Autodesk Inventor part; units mm, degrees
ref_plane "YZ Plane" through (0, 0, 0) normal (1, 0, 0) x (0, 1, 0)
ref_plane "XZ Plane" through (0, 0, 0) normal (0, 1, 0) x (-1, 0, 0)
ref_plane "XY Plane" through (0, 0, 0) normal (0, 0, 1) x (1, 0, 0)
sketch "Sketch1" plane through (0, 0, 0) normal (1, 0, 0) x (0, 1, 0)
  line L0 (0, 0) -> (17.9, 0)
  line L1 (17.9, 0) -> (17.9, 85)
  line L2 (17.9, 85) -> (0, 85)
  line L3 (0, 85) -> (0, 0)
  dimension "d0" = 17.9
  dimension "d1" = 85
extrude "Extrusion1" add sketch "Sketch1" along normal blind 10
fillet "Fillet1" radius 8.95 2 edges at (5, 17.9, 85) (5, 0, 85)
sketch "Sketch2" plane through (10, 0, 0) normal (1, 0, 0) x (0, 0, -1)
  arc A0 (-76.05, 17.9) -> (-76.05, 0) centre (-76.05, 8.95) ccw
  circle A1 centre (-76.05, 8.95) radius 4.75
  point P0 (0, 0)
  dimension "d5" = 9.5
extrude "Extrusion2" cut sketch "Sketch2" against normal blind 10
sketch "Sketch3" plane through (0, 0, 0) normal (0, 0, -1) x (-1, 0, 0)
  line L0 (14.8, 0) -> (-24.8, 0)
  line L1 (-31.8, 7) -> (-31.8, 7)
  line L2 (-24.8, 14) -> (14.8, 14)
  line L3 (21.8, 7) -> (21.8, 7)
  line L4 (0, 0) -> (0, 17.9)
  line L5 (-10, 0) -> (-10, 17.9)
  line L6 (0, 17.9) -> (-10, 17.9)
  circle A0 centre (-25.7, 7) radius 1.6
  circle A1 centre (15.7, 7) radius 1.6
  arc A2 (-24.8, 14) -> (-31.8, 7) centre (-24.8, 7) ccw
  arc A3 (-31.8, 7) -> (-24.8, 0) centre (-24.8, 7) ccw
  arc A4 (21.8, 7) -> (14.8, 14) centre (14.8, 7) ccw
  arc A5 (14.8, 0) -> (21.8, 7) centre (14.8, 7) ccw
  point P0 (21.8, 0)
  point P1 (-31.8, 14)
  point P2 (-31.8, 0)
  point P3 (21.8, 14)
  point P4 (-10, 14)
  point P5 (0, 14)
  point P6 (21.8, 7)
  point P7 (-31.8, 7)
  dimension "d8" = 14
  dimension "d9" = 21.8
  dimension "d10" = 21.8
  dimension "d11" = 17.9
  dimension "d12" = 3.2
  dimension "d13" = 3.2
  dimension "d14" = 6.1
  dimension "d15" = 6.1
  dimension "d16" = 7
  dimension "d17" = 7
  dimension "d23" = 7
extrude "Extrusion3" add sketch "Sketch3" against normal blind 10 contours L0 L4 L2 A4 A5 | L0 L5 L2 L4 | L0 A3 A2 L2 L5
fillet "Fillet3" radius 5.5 2 edges at (10, 7, 10) (0, 7, 10)
fillet "Fillet4" radius 3.9 4 edges at (0, 14, 12.75) (0, 14, 5) (10, 14, 12.75) (10, 14, 5)
sketch "Sketch4" plane through (24.8, 7, 0) normal (0, 0, -1) x (-1, 0, 0)
  line L0 (14.8, 10.9) -> (14.8, -7)
  line L1 (14.8, 10.9) -> (24.8, 10.9)
  line L2 (24.8, 10.9) -> (24.8, 14.4)
  line L3 (19.8, 19.4) -> (19.8, 19.4)
  line L4 (14.8, 14.4) -> (14.8, 10.9)
  circle A0 centre (19.8, 15.7) radius 1.6
  arc A1 (19.8, 19.4) -> (14.8, 14.4) centre (19.8, 14.4) ccw
  arc A2 (24.8, 14.4) -> (19.8, 19.4) centre (19.8, 14.4) ccw
  point P0 (24.8, -7)
  point P1 (24.8, 19.4)
  point P2 (19.8, 19.4)
  dimension "d24" = 8.5
  dimension "d25" = 3.2
  dimension "d26" = 4.8
  dimension "d27" = 5
extrude "Extrusion4" add sketch "Sketch4" against normal blind 10
fillet "Fillet5" radius 3 1 edges at (5, 17.9, 10)
properties part number "Motor Mount V2"
Verification items for the finished model (mm, model axes). A direction names the side the tool comes from. Round coordinates to 2 decimals unless told otherwise and drop trailing zeros. Loops run counter-clockwise (first coordinate to the right, second up) from the corner with the lowest first, then second, coordinate; pieces in that order, holes last. Notation, with made-up numbers: (63.5, 81.25) - (84.5, 81.25) arc R22 ccw to (84.5, 91.25) - close; hole circle Ø5 at (75, 4). An arc over 180 degrees is marked (long way). Answer in a Markdown table with one row per item. Add a question column.
Q1. Section check C-C on y = 7. Enter the section's corners in (x, z) (3 decimals).
Q2. Release check for a two-part mould opening along Y. For faces 4 (the face through (26.97, 6.03, 4.93)), 5 (the face through (5, 8, 0)), 6 (the face through (19, 14, 5)) record: pulls with the +Y half, pulls with the -Y half, needs draft (parallel to the pull), parting line crosses it, or undercut.
Q3. Section check A-A on x = 5. State how many separate pieces and enclosed holes the cut face has, plus the area to 3 significant figures.
Q4. Material ranges on line 1 (Y direction, x = 5, z = 76); line 2 (Z direction, x = 3, y = 9); line 3 (Y direction, x = 15.5, z = 6.5), recorded low to high.
Q5. Section check B-B on z = 75. Enter the section's corners in (x, y).
Q6. Tool access check on faces 1 (the face through (-9, 14, 5)), 2 (the face through (4, 24.3, 10)), 3 (the face through (23.8, 7.1, 10)). Record the directions out of +Z, -Z, +X, -X, +Y, -Y that give a thin tool (end or side, any length) a straight path to the whole face; none if there is none.
Q7. Section check D-D on y = 11. Enter the section's corners in (x, z), plus the area to 3 significant figures.
Q8. Gauge pin test, flat ends, axial feed: pin 1 (5 mm diameter, centred on x = 1, y = 22.5, fed in from -Z); pin 2 (3 mm diameter, centred on x = 7, z = 60.5, fed in from +Y); pin 3 (6.5 mm diameter, centred on y = 5.5, z = 29, fed in from -X); pin 4 (6 mm diameter, centred on y = 12, z = 14, fed in from -X). Record the tip position at first contact, or that the pin passes through.
Found:
| question | item | result |
|---|---|---|
| 1 | outline | (-21.8, 0) - (-17.3, 0) - (-17.3, 10) - (-21.8, 10) - close; (-14.1, 0) - (24.1, 0) - (24.1, 10) - (15.5, 10) arc R5.5 cw to (10, 15.5) - (10, 71.719) - (0, 71.719) - (0, 15.5) arc R5.5 cw to (-5.5, 10) - (-14.1, 10) - close; (0, 80.381) - (10, 80.381) - (10, 84.785) - (0, 84.785) - close; (27.3, 0) - (31.8, 0) - (31.8, 10) - (27.3, 10) - close |
| 2 | face 4 | undercut |
| 2 | face 5 | needs draft |
| 2 | face 6 | pulls with the +Y half |
| 3 | separate pieces | 2 |
| 3 | enclosed holes | 1 |
| 3 | area | 1,470 mm² |
| 4 | line 1 | y = 0 to 4.2, 13.7 to 17.9 |
| 4 | line 2 | z = 0 to 71.3, 80.8 to 85 |
| 4 | line 3 | y = 0 to 14 |
| 5 | outline | (0, 0) - (10, 0) - (10, 4.32) - (0, 4.32) - close; (0, 13.58) - (10, 13.58) - (10, 17.9) - (0, 17.9) - close |
| 6 | face 1 | +Z, -Z, -X, +Y |
| 6 | face 2 | +Z, +X, -X, +Y |
| 6 | face 3 | +Z, +X, +Y, -Y |
| 7 | outline | (-20.54, 0) - (30.54, 0) - (30.54, 10) - (15.5, 10) arc R5.5 cw to (10, 15.5) - (10, 71.77) - (0, 71.77) - (0, 15.5) arc R5.5 cw to (-5.5, 10) - (-20.54, 10) - close; (0, 80.33) - (10, 80.33) - (10, 84.76) - (0, 84.76) - close |
| 7 | area | 1,190 mm² |
| 8 | pin 1 | stops at z = 0 |
| 8 | pin 2 | stops at y = 17.9 |
| 8 | pin 3 | stops at x = 0 |
| 8 | pin 4 | stops at x = -2.34 |
